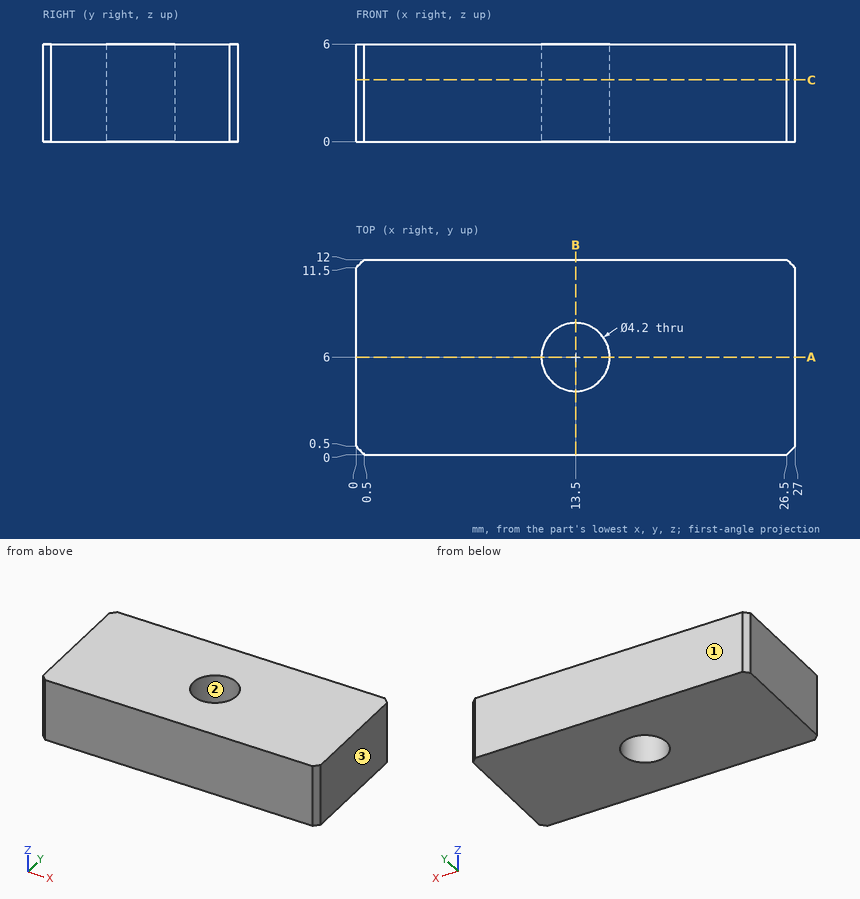
Geometry check sheet. Reference: drawing and pictorial views, mm from the part's lowest x, y, z. Give positions to 0.01 mm unless a question says otherwise; leave off trailing zeros. Order: outer loops, then holes, each group sorted by start corner. A loop starts at its lowest first (then second) coordinate and runs counter-clockwise, first axis right, second up.
1. Thickness scan on L1, parallel to Y at x = 13.5, z = 2.85; L2, parallel to Y at x = 12, z = 2; L3, parallel to X at y = 7.25, z = 4.1. Record the ranges inside material, lowest first.
2. Section check A-A, the plane y = 6. Enter the section's corners in (x, z), and give its area (3 significant figures).
3. Release check for a two-part mould opening along Y. For the marked faces 1, 2 and 3 record: pulls with the +Y half, pulls with the -Y half, needs draft (parallel to the pull), parting line crosses it, or undercut.
4. Section check C-C, the plane z = 3.8. Enter the section's corners in (x, y), and give its area (3 significant figures).
5. Section check B-B, the plane x = 13.5. Enter the section's corners in (y, z).
Values follow:
1. L1: y = 0 to 3.9, 8.1 to 12
1. L2: y = 0 to 4.53, 7.47 to 12
1. L3: x = 0 to 11.81, 15.19 to 27
2. outline: (0, 0) - (11.4, 0) - (11.4, 6) - (0, 6) - close; (15.6, 0) - (27, 0) - (27, 6) - (15.6, 6) - close
2. area: 137 mm2
3. face 1: pulls with the +Y half
3. face 2: undercut
3. face 3: needs draft
4. outline: (0, 0.5) - (0.5, 0) - (26.5, 0) - (27, 0.5) - (27, 11.5) - (26.5, 12) - (0.5, 12) - (0, 11.5) - close; hole circle Ø4.2 at (13.5, 6)
4. area: 310 mm2
5. outline: (0, 0) - (3.9, 0) - (3.9, 6) - (0, 6) - close; (8.1, 0) - (12, 0) - (12, 6) - (8.1, 6) - close
